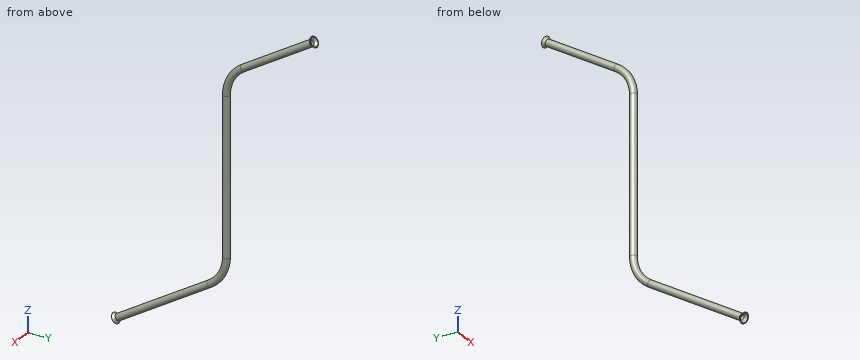
```python
from build123d import *

# Parameters (mm, degrees)
SKETCH1_R           = 2.38125
SKETCH1_R_2         = 1.82245
SKETCH4_R           = 2.38125
SKETCH4_R_2         = 1.82245
SKETCH5_R           = 2.38125
BOSS_EXTRUDE1_DEPTH = 1.778
BOSS_EXTRUDE1_DRAFT = -37
SKETCH6_R           = 1.82245
CUT_EXTRUDE1_DEPTH  = 6.146397849
CUT_EXTRUDE1_DRAFT  = 37
SKETCH7_R           = 2.38125
BOSS_EXTRUDE2_DEPTH = 1.778
BOSS_EXTRUDE2_DRAFT = -37
SKETCH8_R           = 1.82245
CUT_EXTRUDE2_DEPTH  = 6.146397849
CUT_EXTRUDE2_DRAFT  = 37


with BuildPart() as part:
    # Sweep2: sweep along a path in Sketch2
    with BuildLine(Plane(origin=(0, 0, 0), x_dir=(0, 0, -1), z_dir=(1, 0, 0))) as sweep2_path:
        Line((0, 0), (110.130707173, 0))
        ThreePointArc((110.130707173, 0), (122.362068558, -3.138962318), (131.570297464, -11.780015853))
        Line((131.570297464, -11.780015853), (172.430249905, -76.098786725))
    # Sketch1 → Sweep2 (sweep)
    with BuildSketch(Plane.XY):
        Circle(SKETCH1_R)
        Circle(SKETCH1_R_2, mode=Mode.SUBTRACT)
    sweep(path=sweep2_path.line)

    # Sweep3: sweep along a path in Sketch3
    with BuildLine(Plane(origin=(0, 0, 0), x_dir=(0, 0, -1), z_dir=(1, 0, 0))) as sweep3_path:
        Line((-52.084554622, 60.019094007), (-21.439590291, 11.780015853))
        ThreePointArc((-21.439590291, 11.780015853), (-12.231361385, 3.138962318), (0, 0))
    # Sketch4 → Sweep3 (sweep)
    with BuildSketch(Plane.XY):
        Circle(SKETCH4_R)
        Circle(SKETCH4_R_2, mode=Mode.SUBTRACT)
    sweep(path=sweep3_path.line)


with BuildPart() as boss_extrude1_tool:
    # Sketch5 → Boss-Extrude1 (with draft: the straight prism first)
    with BuildSketch(Plane(origin=(0, 66.335772321, 42.141298184), x_dir=(1, 0, 0), z_dir=(0, 0.844078358, 0.536219848))):
        with Locations(Location((0, -11.780015853, 0), (0, 0, 270))):  # turned: the seam where the file's is
            Circle(SKETCH5_R)
    extrude(amount=BOSS_EXTRUDE1_DEPTH)
    # Boss-Extrude1: the draft: its side faces are tilted about the plane it starts from
    boss_extrude1_sides = [boss_extrude1_tool.faces().sort_by_distance(p)[0] for p in [
        (0, 62.046353181, 50.551292477),
    ]]
    draft(boss_extrude1_sides, Plane(origin=(0, 66.335772321, 42.141298184), x_dir=(1, 0, 0), z_dir=(0, 0.844078358, 0.536219848)), BOSS_EXTRUDE1_DRAFT)


with BuildPart() as part_1:
    add(part.part)

    # Boss-Extrude1: add boss_extrude1_tool
    add(boss_extrude1_tool.part)


with BuildPart() as cut_extrude1_tool:
    # Sketch6 → Cut-Extrude1 (with draft: the straight prism first)
    with BuildSketch(Plane(origin=(0, 66.335772321, 42.141298184), x_dir=(1, 0, 0), z_dir=(0, -0.844078358, -0.536219848))):
        with Locations(Location((0, 11.780015853, 0), (0, 0, 90))):  # turned: the seam where the file's is
            Circle(SKETCH6_R)
    extrude(amount=-CUT_EXTRUDE1_DEPTH)
    # Cut-Extrude1: the draft: its side faces are tilted about the plane it starts from
    cut_extrude1_sides = [cut_extrude1_tool.faces().sort_by_distance(p)[0] for p in [
        (0, 63.590348571, 52.194174279),
    ]]
    draft(cut_extrude1_sides, Plane(origin=(0, 66.335772321, 42.141298184), x_dir=(1, 0, 0), z_dir=(0, -0.844078358, -0.536219848)), CUT_EXTRUDE1_DRAFT)


with BuildPart() as part_2:
    add(part_1.part)

    # Cut-Extrude1: cut by cut_extrude1_tool
    add(cut_extrude1_tool.part, mode=Mode.SUBTRACT)


with BuildPart() as boss_extrude2_tool:
    # Sketch7 → Boss-Extrude2 (with draft: the straight prism first)
    with BuildSketch(Plane(origin=(0, -132.261897211, -84.022358583), x_dir=(1, 0, 0), z_dir=(0, -0.844078358, -0.536219848))):
        with Locations(Location((0, -104.738962318, 0), (0, 0, 270))):  # turned: the seam where the file's is
            Circle(SKETCH7_R)
    extrude(amount=BOSS_EXTRUDE2_DEPTH)
    # Boss-Extrude2: the draft: its side faces are tilted about the plane it starts from
    boss_extrude2_sides = [boss_extrude2_tool.faces().sort_by_distance(p)[0] for p in [
        (0, -78.126045899, -170.89698776),
    ]]
    draft(boss_extrude2_sides, Plane(origin=(0, -132.261897211, -84.022358583), x_dir=(1, 0, 0), z_dir=(0, -0.844078358, -0.536219848)), BOSS_EXTRUDE2_DRAFT)


with BuildPart() as part_3:
    add(part_2.part)

    # Boss-Extrude2: add boss_extrude2_tool
    add(boss_extrude2_tool.part)


with BuildPart() as cut_extrude2_tool:
    # Sketch8 → Cut-Extrude2 (with draft: the straight prism first)
    with BuildSketch(Plane(origin=(0, -132.261897211, -84.022358583), x_dir=(1, 0, 0), z_dir=(0, 0.844078358, 0.536219848))):
        with Locations(Location((0, 104.738962318, 0), (0, 0, 90))):  # turned: the seam where the file's is
            Circle(SKETCH8_R)
    extrude(amount=-CUT_EXTRUDE2_DEPTH)
    # Cut-Extrude2: the draft: its side faces are tilted about the plane it starts from
    cut_extrude2_sides = [cut_extrude2_tool.faces().sort_by_distance(p)[0] for p in [
        (0, -79.670041289, -172.539869562),
    ]]
    draft(cut_extrude2_sides, Plane(origin=(0, -132.261897211, -84.022358583), x_dir=(1, 0, 0), z_dir=(0, 0.844078358, 0.536219848)), CUT_EXTRUDE2_DRAFT)


with BuildPart() as part_4:
    add(part_3.part)

    # Cut-Extrude2: cut by cut_extrude2_tool
    add(cut_extrude2_tool.part, mode=Mode.SUBTRACT)


solid = part_4.part
```
Work out the finished part from the listing and answer in its coordinate system (mm). Give positions to 0.01 mm unless a question says otherwise; leave off trailing zeros. Loops run counter-clockwise (first coordinate to the right, second up) from the corner with the lowest first, then second, coordinate; pieces in that order, holes last. Notation, with made-up numbers: M 3,76.25 L 58,76.25 A16 ccw 58,86.25 Z; hole C -11.5,60.25 d1. An arc over 180 degrees is marked long. One line per item, written item: value. Start each with the question number.
1. Each of these flat-tipped pins is pushed along its axis until it touches: P1, Ø4, axis at x = 0, y = 0, coming from the +Z side; P2, Ø4, axis at x = 2, z = -77, coming from the +Y side; P3, Ø1.5, axis at x = 1.5, y = -61, coming from the +Z side. Where does it stop, or does it pass through?
2. Find the intervals of material crossed by probe 1 along Y at (x, z) = (0, -26.5); probe 2 along Y at (x, z) = (0.5, 25.5), in increasing order.
3. Find section B-B (z = -65). Give the vertices of the cut face in (x, y).
Reported:
1. P1: stops at z = 14.97
1. P2: stops at y = 2.38
1. P3: stops at z = -159.92
2. probe 1: y = -2.38 to -1.82, 1.82 to 2.38
2. probe 2: y = 13.83 to 14.9, 21.44 to 22.51
3. outline: C 0,0 d4.76; hole C 0,0 d3.64
